Read the model definition and answer for the solid it produces. Units are mm, in the model's axes. Face numbers are marked on the shaded views. A direction names the side the tool comes from. Round coordinates to 2 decimals unless told otherwise and drop trailing zeros. Loops run counter-clockwise (first coordinate to the right, second up) from the corner with the lowest first, then second, coordinate; pieces in that order, holes last. Notation, with made-up numbers: (65.25, -21.75) - (109.25, -21.75) arc R17 ccw to (109.25, -2.75) - close; hole circle Ø8 at (14, -34.75). An arc over 180 degrees is marked (long way). Answer as CSV lines item,"result".
Autodesk Inventor part; units mm, degrees
ref_plane "YZ Plane" through (0, 0, 0) normal (1, 0, 0) x (0, 1, 0)
ref_plane "XY Plane" through (0, 0, 0) normal (0, 0, 1) x (1, 0, 0)
sketch "Sketch1" plane through (0, 0, 0) normal (0, 0, 1) x (1, 0, 0)
  line L0 (0, 0) -> (5, 0)
  line L1 (5, 0) -> (5, 20)
  line L2 (5, 20) -> (0, 20)
  line L3 (0, 20) -> (0, 0)
  line L4 (5, 12.5) -> (10, 12.5)
  line L5 (10, 12.5) -> (10, 7.5)
  line L6 (10, 7.5) -> (5, 7.5)
  line L7 (5, 7.5) -> (5, 12.5)
  line L8 (0, 10) -> (28.6549, 10) construction
  dimension "d0" = 5
  dimension "d1" = 20
  dimension "d2" = 5
  dimension "d3" = 5
  dimension "d4" = 2.5
extrude "Extrusion1" add sketch "Sketch1" along normal blind 5
ref_plane "Work Plane2" through (0, 10, 0) normal (0, 1, 0) x (-1, 0, 0)
sketch "Sketch2" plane through (0, 10, 0) normal (0, 1, 0) x (-1, 0, 0)
  line L0 (-10, 0) -> (-10, 5)
  line L1 (-10, 2.5) -> (-21, 2.5)
  line L2 (-25, 6.5) -> (-25, 78.5)
  line L3 (-29, 82.5) -> (-40, 82.5)
  arc A0 (-25, 6.5) -> (-21, 2.5) centre (-21, 6.5) ccw
  arc A1 (-25, 78.5) -> (-29, 82.5) centre (-29, 78.5) ccw
  point P0 (0, 0)
  dimension "d11" = 8
  dimension "d12" = 8
  dimension "d13" = 15
  dimension "d14" = 80
  dimension "d16" = 15
sketch "Sketch3" plane through (10, 7.5, 0) normal (1, 0, 0) x (0, 0, -1)
  circle A0 centre (-2.5, 2.5) radius 1.5
  line L0 (0, 5) -> (-5, 5)
  line L1 (0, 0) -> (0, 5)
  point P0 (0, -7.5)
  dimension "d17" = 3
  dimension "d18" = 2.5
  dimension "d19" = 2.5
sweep "Sweep1" add profiles "Sketch3" path "Sketch2" path curves L1 A0 L2 A1 L3
properties part number "gancho"
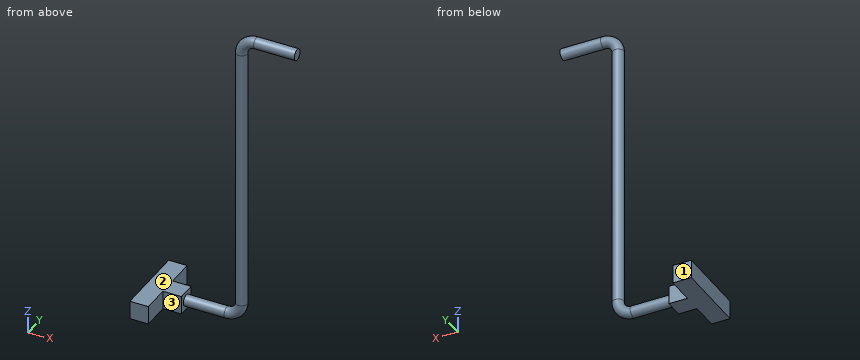
1) A cutting plane is placed at C-C, the plane x = 3. Determine the outline of the cut face in (y, z), plus the area to 3 significant figures.
Entries:
outline,"(0, 0) - (20, 0) - (20, 5) - (0, 5) - close"
area,"100 mm^2"
2) A tool of negligible diameter and unlimited length cuts with its end or side. For the marked faces 1, 2 and 3, from which of +Z, -Z, +X, -X, +Y, -Y can it reach the whole face along a straight path? Write none if from no direction.
Entries:
face 1,"+Z, -Z, +X, -X, +Y"
face 2,"+Z, -X, +Y, -Y"
face 3,"+Z, -Z, +X, -Y"
3) A cutting plane is placed at D-D, the plane y = 16.25. Determine the outline of the cut face in (x, z), plus the area to 3 significant figures.
Entries:
outline,"(0, 0) - (5, 0) - (5, 5) - (0, 5) - close"
area,"25.0 mm^2"
4) Find the intervals of material crossed by line 1 (Z direction, x = 9.5, y = 7.75); line 2 (X direction, y = 9.25, z = 25); line 3 (Z direction, x = 31, y = 9.5), in increasing order.
Entries:
line 1,"z = 0 to 5"
line 2,"x = 23.7 to 26.3"
line 3,"z = 81.09 to 83.91"
5) A cutting plane is placed at B-B, the plane z = 56.5. Determine the outline of the cut face in (x, y), plus the area to 3 significant figures.
Entries:
outline,"circle Ø3 at (25, 10)"
area,"7.07 mm^2"
6) A cutting plane is placed at A-A, the plane y = 10. Determine the outline of the cut face in (x, z).
Entries:
outline,"(0, 0) - (10, 0) - (10, 1) - (21, 1) arc R5.5 ccw to (26.5, 6.5) - (26.5, 78.5) arc R2.5 cw to (29, 81) - (40, 81) - (40, 84) - (29, 84) arc R5.5 ccw to (23.5, 78.5) - (23.5, 6.5) arc R2.5 cw to (21, 4) - (10, 4) - (10, 5) - (0, 5) - close"
7) Each of these flat-tipped pins is pushed along its axis until it touches: P1, Ø1.5, axis at y = 5.5, z = 3.5, coming from the +X side; P2, Ø8, axis at x = 8, y = 16, coming from the +Z side; P3, Ø2.5, axis at x = 8.5, z = 3, coming from the +Y side; P4, Ø12, axis at x = 13, y = 9.5, coming from the -Z side. Where does it stop, or does it pass through?
Entries:
P1,"stops at x = 5"
P2,"stops at z = 5"
P3,"stops at y = 12.5"
P4,"stops at z = 0"
